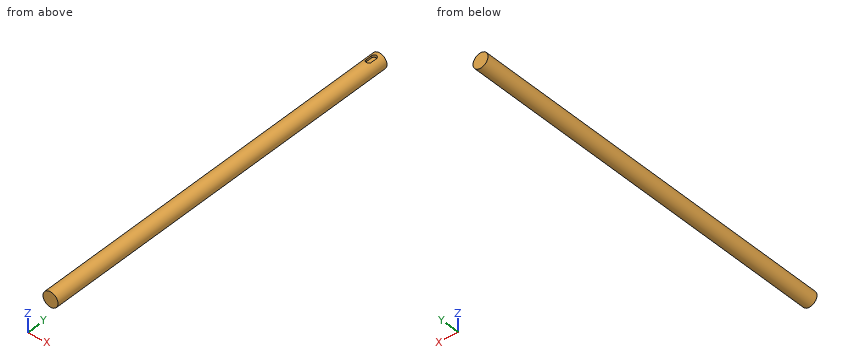
from build123d import *

# Parameters (mm, degrees)
F0_R     = 6
F1_DEPTH = 300
F4_DEPTH = 4


with BuildPart() as f1:
    # F0 (on Front) → F1 (new body)
    with BuildSketch(Plane.XZ):
        Circle(F0_R)
    extrude(amount=F1_DEPTH)

    # F3 (on offset) → F4 (cut)
    with BuildSketch(Plane.XY.offset(8)):
        with BuildLine():
            Line((-2, -5), (-2, -10))
            ThreePointArc((-2, -10), (0, -12), (2, -10))
            Line((2, -10), (2, -5))
            ThreePointArc((2, -5), (0, -3), (-2, -5))
        make_face()
    extrude(amount=-F4_DEPTH, mode=Mode.SUBTRACT)


solid = f1.part
The listing builds one solid part. Answer for the finished solid, in the listing's coordinates (mm). Give positions to 0.01 mm unless a question says otherwise; leave off trailing zeros. Order: outer loops, then holes, each group sorted by start corner. A loop starts at its lowest first (then second) coordinate and runs counter-clockwise, first axis right, second up. Notation, with made-up numbers: (80, 88) - (99, 88) arc R32 ccw to (99, 119) - close; hole circle Ø3 at (-29.5, 85.5). An arc over 180 degrees is marked (long way). One line per item, written item: value. Start each with the question number.
1) A cutting plane is placed at B-B on y = -137.5. Give the vertices of the cut face in (x, z).
2) A cutting plane is placed at A-A on x = -4. Give the vertices of the cut face in (y, z), then the cut area to 3 significant figures.
3) Find the intervals of material crossed by L1, parallel to X at y = -227, z = -0.25; L2, parallel to X at y = -97.5, z = -3, in increasing order.
4) Given pin 1 Ø1 at (x, z) = (4.5, -4) entering from -Y; pin 2 Ø3 at (y, z) = (-156, 4.5) entering from -X; pin 3 Ø0.5 at (y, z) = (-8, 5) entering from -X; pin 4 Ø6 at (x, y) = (3.5, -196.5) entering from +Z, each flat-ended and moving along its own axis, determine where each tip first touches the part or whether it passes through.
5) A cutting plane is placed at C-C on z = -3. Give the vertices of the cut face in (x, y).
Answer sheet:
1. outline: circle Ø12 at (0, 0)
2. outline: (-300, -4.47) - (0, -4.47) - (0, 4.47) - (-300, 4.47) - close
2. area: 2,680 mm2
3. L1: x = -5.99 to 5.99
3. L2: x = -5.2 to 5.2
4. pin 1: stops at y = -300
4. pin 2: stops at x = -5.2
4. pin 3: stops at x = -3.67
4. pin 4: stops at z = 5.98
5. outline: (-5.2, -300) - (5.2, -300) - (5.2, 0) - (-5.2, 0) - close
